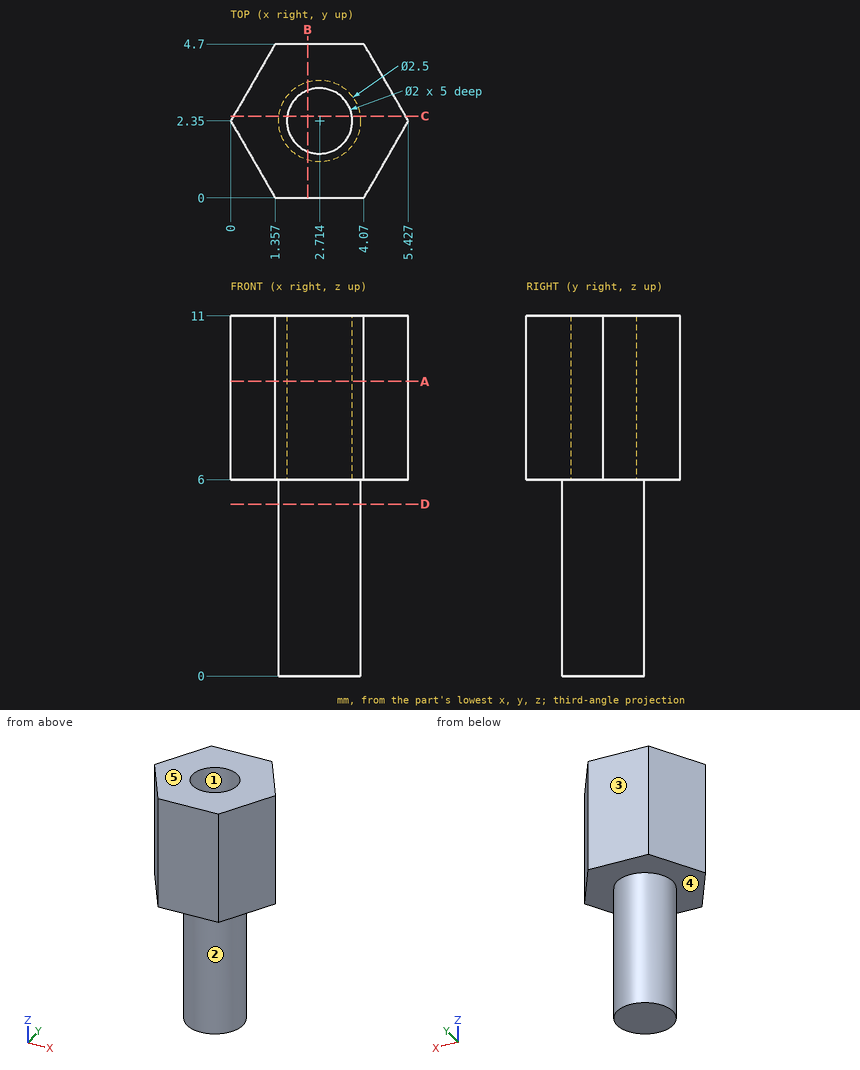
Here's the drawing with two shaded views (mm, measured from the low corner). I have some questions. A direction names the side the tool comes from. Give positions to 0.01 mm unless a question says otherwise; leave off trailing zeros. Loops run counter-clockwise (first coordinate to the right, second up) from the corner with the lowest first, then second, coordinate; pieces in that order, holes last. Notation, with made-up numbers: (53, 78.5) - (79, 78.5) arc R15 ccw to (79, 91.5) - close; hole circle Ø8 at (75.5, 34.5). An arc over 180 degrees is marked (long way). Answer in a Markdown table with one row per item. Add a question column.
Q1. If we section it at C-C (y = 2.5): List the corners of the cut face in (x, z) for me (1 decimal).
Q2. Which directions (+Z, -Z, +X, -X, +Y, -Y) give clear straight access to the entire face, cutting with the end or side of a thin tool? Please do the marked faces 4 and 5.
Q3. Please list where these lines run through material, in increasing order: L1, parallel to Z at x = 3.85, y = 1.75; L2, parallel to X at y = 2.1, z = 10.75 (1 decimal); L3, parallel to Y at x = 2.3, z = 3. Write a range as from..to.
Q4. We'd pull the mould along X, two halves only. Please class the marked faces 1, 2 and 3: +X half, -X half, draft (parallel to the pull), parting line (faces both ways), or undercut.
Q5. If we section it at A-A (z = 9): List the corners of the cut face in (x, y) for me, plus the area to 3 significant figures.
Q6. If we section it at B-B (x = 2.35): List the corners of the cut face in (y, z) for me.
Q7. If we section it at D-D (z = 5.25): List the corners of the cut face in (x, y) for me.
Q8. For pin 1 (1 mm diameter, centred on x = 2.5, z = 4.5, fed in from -Y), with a flat end and sliding along its axis, tell me the tip position at first contact or that it passes through.
The answers:
| question | item | result |
|---|---|---|
| 1 | outline | (0.1, 6) - (1.5, 6) - (1.5, 0) - (4, 0) - (4, 6) - (5.3, 6) - (5.3, 11) - (3.7, 11) - (3.7, 6) - (1.7, 6) - (1.7, 11) - (0.1, 11) - close |
| 2 | face 4 | -Z |
| 2 | face 5 | +Z, +X, -X, +Y, -Y |
| 3 | L1 | z = 6..11 |
| 3 | L2 | x = 0.1..1.7, 3.7..5.3 |
| 3 | L3 | y = 1.17..3.53 |
| 4 | face 1 | undercut |
| 4 | face 2 | parting line |
| 4 | face 3 | draft |
| 5 | outline | (0, 2.35) - (1.36, 0) - (4.07, 0) - (5.43, 2.35) - (4.07, 4.7) - (1.36, 4.7) - close; hole circle Ø2 at (2.71, 2.35) |
| 5 | area | 16.0 mm^2 |
| 6 | outline | (0, 6) - (1.15, 6) - (1.15, 0) - (3.55, 0) - (3.55, 6) - (4.7, 6) - (4.7, 11) - (3.28, 11) - (3.28, 6) - (1.42, 6) - (1.42, 11) - (0, 11) - close |
| 7 | outline | circle Ø2.5 at (2.71, 2.35) |
| 8 | pin 1 | stops at y = 1.1 |
